The model under review builds one solid part; all positions refer to its coordinate system, in mm. A direction names the side the tool comes from. Round coordinates to 2 decimals unless told otherwise and drop trailing zeros. Write each loop counter-clockwise with the first axis right and the second up, starting at its lowest first coordinate (ties: lowest second). Pieces come first, ordered by that corner, then holes. Notation, with made-up numbers: M 16,-16.75 L 21,-16.75 A16 cw 21,-6.75 Z; hole C 44.25,10.25 d8. An arc over 180 degrees is marked long. One line per item, written item: value. Start each with the question number.
1) Take a section at C-C, the plane z = 5. Write out the cut boundary in (x, y).
2) Mouldability with a two-part tool opening along Z and no side actions: class faces 3 (the face through (0, -1, -7)), 4 (the face through (0, 2, -9.25)), 5 (the face through (1.88, -0.51, 5.96)) as +Z half, -Z half, draft (parallel to the pull), parting line (faces both ways), or undercut.
3) Wall thickness on probe 1 along Z at (x, y) = (0, -0.4); probe 2 along X at (y, z) = (5, 1.25); probe 3 along X at (y, z) = (2, 0.25): over which ranges is each line inside the solid? List them lowest first.
4) Take a section at D-D, the plane x = -10.75. Write out the cut boundary in (y, z), and give its area (3 significant figures).
5) Tool access review of faces 1 (the face through (-2.777, 2.958, 6.697)), 2 (the face through (-8.65, 1.38, -0.28)): name each direction out of +Z, -Z, +X, -X, +Y, -Y from which nothing blocks a thin tool from reaching the whole face with its end or side.
6) For P1, Ø10, axis at x = 0, z = 0, coming from the +Y side; P2, Ø8, axis at x = 3, z = -6, coming from the +Y side; P3, Ø6.5, axis at x = -10.75, z = 0, coming from the -Y side; P4, Ø3, axis at x = 9.5, y = 1.5, coming from the +Z side, all flat-tipped, find the tip position at first contact; note any pin that passes through.
7) Take a section at B-B, the plane y = -0.5. Write out the cut boundary in (x, z).
8) Take a section at A-A, the plane x = 0. Write out the cut boundary in (y, z), and give its area (3 significant figures).
from build123d import *

# Parameters (mm, degrees)
SKETCH1_R           = 2
SKETCH1_R_2         = 7.25
BOSS_EXTRUDE1_DEPTH = 6
BOSS_EXTRUDE2_START = -1
SKETCH1_3_R         = 2
SKETCH1_3_R_2       = 7.25
SKETCH1_3_R_3       = 6.25
BOSS_EXTRUDE2_DEPTH = 1
CHAMFER1_SIZE       = 2.5


with BuildPart() as part:
    # Sketch1 → Boss-Extrude1 (new body)
    with BuildSketch(Plane(origin=(0, 0, 0), x_dir=(1, 0, 0), z_dir=(0, 1, 0))):
        with BuildLine():
            Line((-5.5, -9.25), (5.5, -9.25))
            ThreePointArc((5.5, -9.25), (14.75, 0), (5.5, 9.25))
            Line((5.5, 9.25), (-5.5, 9.25))
            ThreePointArc((-5.5, 9.25), (-14.75, 0), (-5.5, -9.25))
        make_face()
        with Locations(Location((10.75, 0, 0), (0, 0, 270))):
            Circle(SKETCH1_R, mode=Mode.SUBTRACT)
        with Locations(Location((0, 0, 0), (0, 0, 270))):
            Circle(SKETCH1_R_2, mode=Mode.SUBTRACT)
        with Locations(Location((-10.75, 0, 0), (0, 0, 270))):
            Circle(SKETCH1_R, mode=Mode.SUBTRACT)
    extrude(amount=BOSS_EXTRUDE1_DEPTH)

    # Sketch1<3> → Boss-Extrude2 (add)
    # profile 1 of 2: a face of its own
    with BuildSketch(Plane(origin=(0, 0, 0), x_dir=(1, 0, 0), z_dir=(0, 1, 0)).offset(BOSS_EXTRUDE2_START)):
        with BuildLine():
            Line((-5.5, -9.25), (5.5, -9.25))
            ThreePointArc((5.5, -9.25), (14.75, 0), (5.5, 9.25))
            Line((5.5, 9.25), (-5.5, 9.25))
            ThreePointArc((-5.5, 9.25), (-14.75, 0), (-5.5, -9.25))
        make_face()
        with Locations(Location((10.75, 0, 0), (0, 0, 270))):
            Circle(SKETCH1_3_R, mode=Mode.SUBTRACT)
        with Locations(Location((0, 0, 0), (0, 0, 270))):
            Circle(SKETCH1_3_R_2, mode=Mode.SUBTRACT)
        with Locations(Location((-10.75, 0, 0), (0, 0, 270))):
            Circle(SKETCH1_3_R, mode=Mode.SUBTRACT)
    # profile 2 of 2: a face of its own
    with BuildSketch(Plane(origin=(0, 0, 0), x_dir=(1, 0, 0), z_dir=(0, 1, 0)).offset(BOSS_EXTRUDE2_START)):
        with Locations(Location((0, 0, 0), (0, 0, 270))):
            Circle(SKETCH1_3_R_2)
        with Locations(Location((0, 0, 0), (0, 0, 270))):
            Circle(SKETCH1_3_R_3, mode=Mode.SUBTRACT)
    extrude(amount=BOSS_EXTRUDE2_DEPTH)

    # Chamfer1
    # the kernel refuses this chamfer: 2.5 mm, written as the material it takes off along each edge
    with BuildSketch(Plane(origin=(10.75, -1, 0), x_dir=(0, 0, 1), z_dir=(-1, 0, 0))) as chamfer1_piece_1:
        Polygon((2 + CHAMFER1_SIZE, 0), (2, CHAMFER1_SIZE), (2, 0), align=None)
    revolve(axis=Axis((10.75, -1, 0), (0, 1, 0)), mode=Mode.SUBTRACT)
    with BuildSketch(Plane(origin=(-10.75, -1, 0), x_dir=(0, 0, 1), z_dir=(-1, 0, 0))) as chamfer1_piece_2:
        Polygon((2 + CHAMFER1_SIZE, 0), (2, CHAMFER1_SIZE), (2, 0), align=None)
    revolve(axis=Axis((-10.75, -1, 0), (0, 1, 0)), mode=Mode.SUBTRACT)


solid = part.part
Checked values:
1. outline: M -13.28,-1 L -3.75,-1 L -3.75,0 L -5.25,0 L -5.25,6 L -13.28,6 Z; M 3.75,-1 L 13.28,-1 L 13.28,6 L 5.25,6 L 5.25,0 L 3.75,0 Z
2. face 3: draft
2. face 4: -Z half
2. face 5: undercut
3. probe 1: z = -9.25 to -6.25, 6.25 to 9.25
3. probe 2: x = -14.67 to -12.31, -9.19 to -7.14, 7.14 to 9.19, 12.31 to 14.67
3. probe 3: x = -14.75 to -12.73, -8.77 to -7.25, 7.25 to 8.77, 12.73 to 14.75
4. outline: M -1,-7.62 L 6,-7.62 L 6,-2 L 1.5,-2 L -1,-4.5 Z; M -1,4.5 L 1.5,2 L 6,2 L 6,7.62 L -1,7.62 Z
4. area: 72.4 mm2
5. face 1: +Y
5. face 2: -Y
6. P1: passes through
6. P2: stops at y = 6
6. P3: stops at y = 0.25
6. P4: stops at z = 8.91
7. outline: M -5.5,-9.25 L 5.5,-9.25 A9.25 ccw 5.5,9.25 L -5.5,9.25 A9.25 ccw Z; hole C -10.75,0 d8; hole C 0,0 d12.5; hole C 10.75,0 d8
8. outline: M -1,-9.25 L 6,-9.25 L 6,-7.25 L 0,-7.25 L 0,-6.25 L -1,-6.25 Z; M -1,6.25 L 0,6.25 L 0,7.25 L 6,7.25 L 6,9.25 L -1,9.25 Z
8. area: 30.0 mm2
